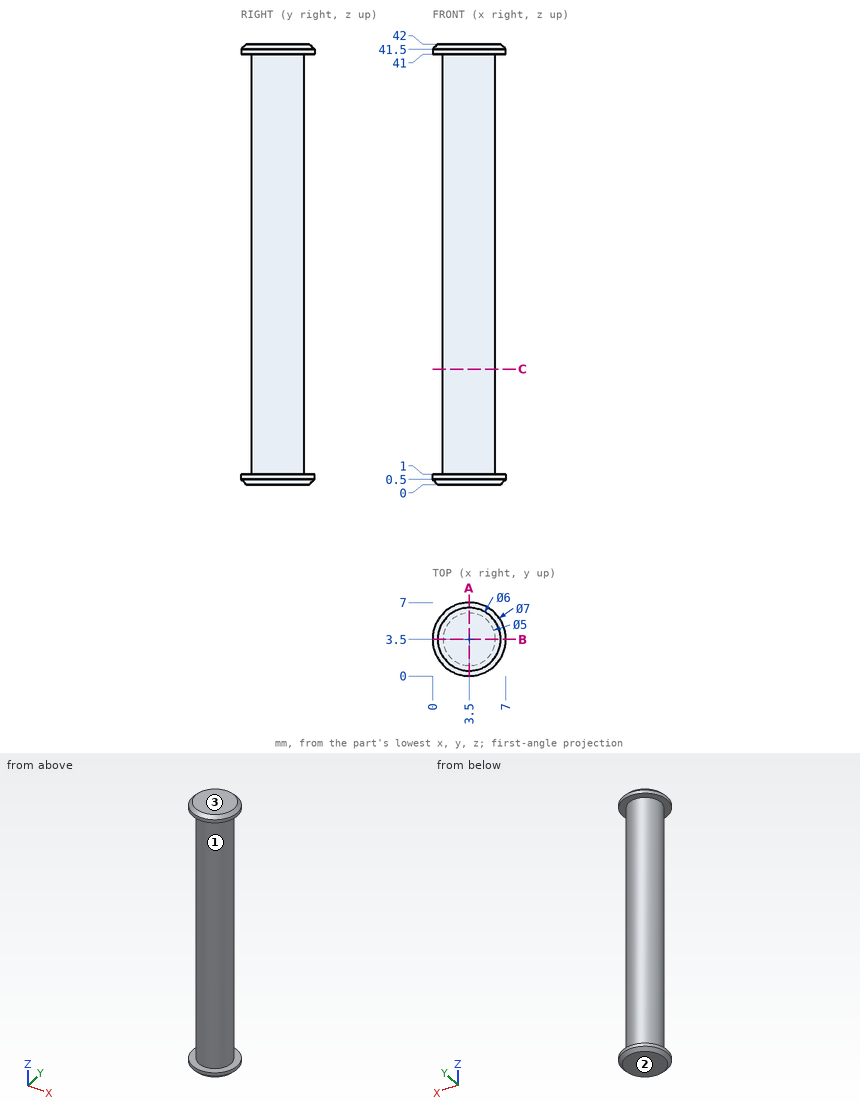
Could you check a few things on this drawing? It's one solid part, dimensions in mm from its lowest x, y, z. Coordinates: 2 decimals unless noted, no trailing zeros. Order: outer loops, then holes, each group sorted by start corner. A loop starts at its lowest first (then second) coordinate and runs counter-clockwise, first axis right, second up. Notation, with made-up numbers: M 56,-16 L 86,-16 A6 ccw 86,-7 Z; hole C -36,6.25 d2. An arc over 180 degrees is marked long. Use a Markdown table: item, result. Add a question column.
Q1. We'd pull the mould along Z, two halves only. Please class the marked faces 1, 2 and 3: pulls with the +Z half, pulls with the -Z half, needs draft (parallel to the pull), parting line crosses it, or undercut.
Q2. I want a section at A-A on x = 3.5. List the corners of the cut face in (y, z) for me.
Q3. If I drill on L1, parallel to Z at x = 1, y = 2; L2, parallel to Z at x = 0.5, y = 2.75; L3, parallel to Y at x = 3.75, z = 17, over which ranges is the centre line in solid material (lowest first)?
Q4. I want a section at C-C on z = 11. List the corners of the cut face in (x, y) for me, then the cut area to 3 significant figures.
Q5. I'm going to push flat-ended pins straight in: pin 1 (4 mm diameter, centred on y = 5, z = 35, fed in from -X); pin 2 (1 mm diameter, centred on x = 4.5, z = 9.5, fed in from +Y); pin 3 (1 mm diameter, centred on y = 4.5, z = 27, fed in from -X). Where does each tip first touch, or does it pass through?
Checked values:
| question | item | result |
|---|---|---|
| 1 | face 1 | undercut |
| 1 | face 2 | pulls with the -Z half |
| 1 | face 3 | pulls with the +Z half |
| 2 | outline | M 0,0.5 L 0.5,0 L 6.5,0 L 7,0.5 L 7,1 L 6,1 L 6,41 L 7,41 L 7,41.5 L 6.5,42 L 0.5,42 L 0,41.5 L 0,41 L 1,41 L 1,1 L 0,1 Z |
| 3 | L1 | 0 to 1, 41 to 42 |
| 3 | L2 | 0.09 to 1, 41 to 41.91 |
| 3 | L3 | 1.01 to 5.99 |
| 4 | outline | C 3.5,3.5 d5 |
| 4 | area | 19.6 mm² |
| 5 | pin 1 | x = 1 |
| 5 | pin 2 | y = 5.95 |
| 5 | pin 3 | x = 1.05 |
